Model file for the job. Use its own axes, mm. Face numbers are marked on the shaded views. A direction names the side the tool comes from. Round coordinates to 2 decimals unless told otherwise and drop trailing zeros. Write each loop counter-clockwise with the first axis right and the second up, starting at its lowest first coordinate (ties: lowest second). Pieces come first, ordered by that corner, then holes. Notation, with made-up numbers: (89, 18.25) - (148, 18.25) arc R20 cw to (148, 23.25) - close; hole circle Ø1 at (73.5, 27). An arc over 180 degrees is marked (long way). One line per item, written item: value.
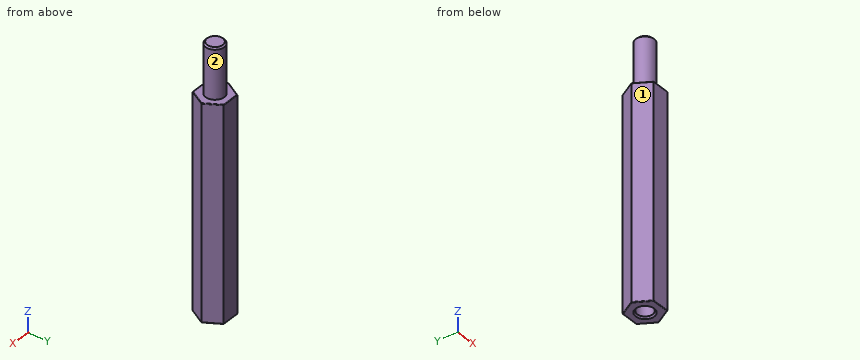
from build123d import *

# Parameters (mm, degrees)
SKETCH_1_R      = 1.5
EXTRUDE_1_DEPTH = 8
EXTRUDE_3_DEPTH = 34
M3X0_51_D       = 2.5
M3X0_51_DEPTH   = 4.3
M3X0_51_TIP     = 0.751075774
CHAMFER_1_SIZE  = 0.25
FILLET_1_R      = 0.1


with BuildPart() as part:
    # Эскиз1 → Бобышка-Вытянуть1 (new body)
    with BuildSketch(Plane.XY):
        Circle(SKETCH_1_R)
    extrude(amount=EXTRUDE_1_DEPTH)

    # Эскиз3 → Бобышка-Вытянуть3 (add)
    with BuildSketch(Plane(origin=(0, 0, 0), x_dir=(-1, 0, 0), z_dir=(0, 0, -1))):
        Polygon((2.886751346, 0), (1.443375673, 2.5), (-1.443375673, 2.5), (-2.886751346, 0), (-1.443375673, -2.5), (1.443375673, -2.5), align=None)
    extrude(amount=EXTRUDE_3_DEPTH)

    # Сверление под метчик M3x0.51
    with Locations(Plane(origin=(0, 0, -34), x_dir=(-1, 0, 0), z_dir=(0, 0, -1))):
        with Locations((0, 0)):
            Hole(M3X0_51_D / 2, depth=M3X0_51_DEPTH)
            with Locations((0, 0, -(M3X0_51_DEPTH + M3X0_51_TIP / 2))):  # 118° drill point
                Cone(0, M3X0_51_D / 2, M3X0_51_TIP, mode=Mode.SUBTRACT)

    # Фаска1
    chamfer_1_edges = [part.edges().sort_by_distance(p)[0] for p in [
        (-1.25, 0, -34),
        (-1.5, 0, 8),
    ]]
    chamfer(chamfer_1_edges, length=CHAMFER_1_SIZE)

    # Скругление1
    fillet_1_edges = [part.edges().sort_by_distance(p)[0] for p in [
        (-2.165063509, -1.25, 0),
        (-1.443375673, -2.5, -17),
        (-2.165063509, 1.25, 0),
        (-2.886751346, 0, -17),
        (0, 2.5, 0),
        (-1.443375673, 2.5, -17),
        (2.165063509, 1.25, 0),
        (1.443375673, 2.5, -17),
        (2.165063509, -1.25, 0),
        (2.886751346, 0, -17),
        (0, -2.5, 0),
        (1.443375673, -2.5, -17),
        (-2.165063509, -1.25, -34),
        (-2.165063509, 1.25, -34),
        (0, 2.5, -34),
        (2.165063509, 1.25, -34),
        (2.165063509, -1.25, -34),
        (0, -2.5, -34),
    ]]
    fillet(fillet_1_edges, radius=FILLET_1_R)


solid = part.part
1. Band-saw the part on A-A on z = -0.5. Write the cut outline in (x, y).
Report:
outline: (-2.86, -0.05) - (-1.47, -2.45) arc R0.1 ccw to (-1.39, -2.5) - (1.39, -2.5) arc R0.1 ccw to (1.47, -2.45) - (2.86, -0.05) arc R0.1 ccw to (2.86, 0.05) - (1.47, 2.45) arc R0.1 ccw to (1.39, 2.5) - (-1.39, 2.5) arc R0.1 ccw to (-1.47, 2.45) - (-2.86, 0.05) arc R0.1 ccw to start
2. Drop a flat-ended pin along its axis: pin 1 (1 mm diameter, centred on y = 1.5, z = -7, fed in from +X). Give the stop position or say it passes through.
Report:
pin 1: x = 2.31
3. Wall check: probe 1 along Y at (x, z) = (0, -31.3); probe 2 along X at (y, z) = (0, -31.35); probe 3 along Z at (x, y) = (-1, -1.45). Give the ranges that are in metal, low to high. Write a range as [from, to].
Report:
probe 1: [-2.5, -1.25], [1.25, 2.5]
probe 2: [-2.87, -1.25], [1.25, 2.87]
probe 3: [-34, 0]
4. Tool access for the marked faces 1 and 2: list every direction of +Z, -Z, +X, -X, +Y, -Y with a clear straight run to the whole face (end or side of a thin tool).
Report:
face 1: +Z, -Z, -X, -Y
face 2: +Z
